```python
from build123d import *

# Parameters (mm, degrees)
SKETCH_1_W          = 300
SKETCH_1_H          = 300
EXTRUDE_3_DEPTH     = 200
SKETCH_5_R          = 32.35
CUT_EXTRUDE_3_DEPTH = 62
SKETCH_6_R          = 38.24
CUT_EXTRUDE_4_DEPTH = 23.7
CUT_EXTRUDE_5_REACH = 392.512
SKETCH_8_W          = 75.602160899
SKETCH_8_H          = 50
SKETCH_10_R         = 1.35
CUT_EXTRUDE_7_DEPTH = 5
FILLET_1_R          = 10


with BuildPart() as part:
    # 草图1 → 凸台-拉伸3 (new body)
    with BuildSketch(Plane.XY):
        Rectangle(SKETCH_1_W, SKETCH_1_H)
    extrude(amount=EXTRUDE_3_DEPTH)

    # 草图5 → 切除-拉伸3 (cut)
    with BuildSketch(Plane(origin=(0, 0, 0), x_dir=(-1, 0, 0), z_dir=(0, 0, -1))):
        Circle(SKETCH_5_R)
    extrude(amount=-CUT_EXTRUDE_3_DEPTH, mode=Mode.SUBTRACT)

    # 草图6 → 切除-拉伸4 (cut)
    with BuildSketch(Plane(origin=(0, 0, 0), x_dir=(-1, 0, 0), z_dir=(0, 0, -1))):
        Circle(SKETCH_6_R)
    extrude(amount=-CUT_EXTRUDE_4_DEPTH, mode=Mode.SUBTRACT)

    # 草图8 → 切除-拉伸5 (cut, up to next)
    with BuildSketch(Plane.ZY.offset(150), mode=Mode.PRIVATE) as cut_extrude_5_sk1:
        with Locations((85.011080449, 0)):
            Rectangle(SKETCH_8_W, SKETCH_8_H)
    cut_extrude_5_tool1 = extrude(cut_extrude_5_sk1.sketch, amount=-CUT_EXTRUDE_5_REACH, mode=Mode.PRIVATE) & part.part
    add(cut_extrude_5_tool1.solids().sort_by_distance((-150, 0, 85.01108))[0], mode=Mode.SUBTRACT)

    # 草图10 → 切除-拉伸7 (cut)
    with BuildSketch(Plane(origin=(0, 0, 23.7), x_dir=(-1, 0, 0), z_dir=(0, 0, -1))):
        with Locations((0, -35.295)):
            Circle(SKETCH_10_R)
        with Locations((-14.355769817, -32.243586927)):
            Circle(SKETCH_10_R)
        with Locations((-26.229296615, -23.616964751)):
            Circle(SKETCH_10_R)
        with Locations((-33.567539743, -10.906754816)):
            Circle(SKETCH_10_R)
        with Locations((-35.101650297, 3.689332111)):
            Circle(SKETCH_10_R)
        with Locations((-30.566366627, 17.6475)):
            Circle(SKETCH_10_R)
        with Locations((-20.74588048, 28.554254816)):
            Circle(SKETCH_10_R)
        with Locations((-7.338243127, 34.523719568)):
            Circle(SKETCH_10_R)
        with Locations((7.338243127, 34.523719568)):
            Circle(SKETCH_10_R)
        with Locations((20.74588048, 28.554254816)):
            Circle(SKETCH_10_R)
        with Locations((30.566366627, 17.6475)):
            Circle(SKETCH_10_R)
        with Locations((35.101650297, 3.689332111)):
            Circle(SKETCH_10_R)
        with Locations((33.567539743, -10.906754816)):
            Circle(SKETCH_10_R)
        with Locations((26.229296615, -23.616964751)):
            Circle(SKETCH_10_R)
        with Locations((14.355769817, -32.243586927)):
            Circle(SKETCH_10_R)
    extrude(amount=-CUT_EXTRUDE_7_DEPTH, mode=Mode.SUBTRACT)

    # 圆角1
    fillet_1_edges = [part.edges().sort_by_distance(p)[0] for p in [
        (0, -150, 200),
        (150, -150, 100),
        (-150, -150, 100),
        (-150, 150, 100),
        (150, 150, 100),
    ]]
    fillet(fillet_1_edges, radius=FILLET_1_R)


solid = part.part
```
Work out the finished part from the listing and answer in its coordinate system (mm). A direction names the side the tool comes from. Round coordinates to 2 decimals unless told otherwise and drop trailing zeros. Write each loop counter-clockwise with the first axis right and the second up, starting at its lowest first coordinate (ties: lowest second). Pieces come first, ordered by that corner, then holes. Notation, with made-up numbers: (-10, 31.5) -> (36, 31.5) arc R22 cw to (36, 60.5) -> close; hole circle Ø4 at (-40, 51). An arc over 180 degrees is marked (long way). Write each question's results on one line, items separated by ' | '.
1) For a pull along X with two mould halves and no side action, classify faces 4 (the flat face through (-86, 0, 47.21)), 5 (the cylindrical face through (-147.15, -146.99, 101.4)), 6 (the flat face through (31.34, 8.68, 23.7)) as +X half, -X half, draft (parallel to the pull), parting line (faces both ways), or undercut.
Findings:
face 4: draft | face 5: -X half | face 6: undercut
2) Which of the six approach directions +Z, -Z, +X, -X, +Y, -Y give full straight-line access (tool end or side, diameter ignored) to faces 1 (the cylindrical face through (146.99, 147.15, 101.4)), 2 (the flat face through (-2, 25, 84)), 3 (the flat face through (0, -28, 62))?
Findings:
face 1: +Z, -Z, +X, +Y | face 2: +X, -X | face 3: -Z
3) Flat-ended cylindrical pins translate along their axes: pin 1 (1.4 mm diameter, centred on x = 0, y = -35, fed in from -Z); pin 2 (4.5 mm diameter, centred on x = 26.23, y = -23.62, fed in from -Z); pin 3 (23 mm diameter, centred on x = -17, y = -5.5, fed in from -Z). Find the tip coordinate at first contact, or state that the pin passes through.
Findings:
pin 1: stops at z = 28.7 | pin 2: stops at z = 23.7 | pin 3: stops at z = 122.81
4) Consider line 1 along Z through (x, y) = (137.5, 0); line 2 along Y through (x, z) = (22, 56); line 3 along Y through (x, z) = (-14.5, 40). Determine where each line is inside the solid, lowest interval first. Write a range as [from, to].
Findings:
line 1: z = [0, 47.21], [122.81, 200] | line 2: y = [-150, -25], [25, 150] | line 3: y = [-150, -28.92], [28.92, 150]
5) The part is cut by section A-A (z = 91). Write down the section's boundary in (x, y), and give its area (3 significant figures).
Findings:
outline: (-150, -140) arc R10 ccw to (-140, -150) -> (140, -150) arc R10 ccw to (150, -140) -> (150, -25) -> (-150, -25) -> close; (-150, 25) -> (150, 25) -> (150, 140) arc R10 ccw to (140, 150) -> (-140, 150) arc R10 ccw to (-150, 140) -> close | area: 74,900 mm²
6) The part is cut by section D-D (z = 55). Write down the section's boundary in (x, y).
Findings:
outline: (-150, -140) arc R10 ccw to (-140, -150) -> (140, -150) arc R10 ccw to (150, -140) -> (150, -25) -> (20.53, -25) arc R32.35 cw to (-20.53, -25) -> (-150, -25) -> close; (-150, 25) -> (-20.53, 25) arc R32.35 cw to (20.53, 25) -> (150, 25) -> (150, 140) arc R10 ccw to (140, 150) -> (-140, 150) arc R10 ccw to (-150, 140) -> close
7) The part is cut by section C-C (z = 13). Write down the section's boundary in (x, y), and give its area (3 significant figures).
Findings:
outline: (-150, -140) arc R10 ccw to (-140, -150) -> (140, -150) arc R10 ccw to (150, -140) -> (150, 140) arc R10 ccw to (140, 150) -> (-140, 150) arc R10 ccw to (-150, 140) -> close; hole circle Ø76.48 at (0, 0) | area: 85,300 mm²
8) The part is cut by section B-B (x = 115). Write down the section's boundary in (y, z).
Findings:
outline: (-150, 0) -> (150, 0) -> (150, 200) -> (-140, 200) arc R10 ccw to (-150, 190) -> close; hole (-25, 47.21) -> (25, 47.21) -> (25, 122.81) -> (-25, 122.81) -> close
